from build123d import *

# Parameters (mm, degrees)
ESQUISSE1_W        = 149.75
ESQUISSE1_H        = 135
ESQUISSE1_R        = 1.75
ESQUISSE1_W_2      = 45.5
ESQUISSE1_H_2      = 24.5
BOSS_EXTRU_1_DEPTH = 3
CONG_1_R           = 5
CONG_2_R           = 1


with BuildPart() as part:
    # Esquisse1 → Boss.-Extru.1 (new body)
    with BuildSketch(Plane.XY):
        Rectangle(ESQUISSE1_W, ESQUISSE1_H)
        with Locations((-70, 62.5)):
            Circle(ESQUISSE1_R, mode=Mode.SUBTRACT)
        with Locations((70, 62.5)):
            Circle(ESQUISSE1_R, mode=Mode.SUBTRACT)
        with Locations((55, -51.5)):
            Circle(ESQUISSE1_R, mode=Mode.SUBTRACT)
        with Locations((-55, -51.5)):
            Circle(ESQUISSE1_R, mode=Mode.SUBTRACT)
        with Locations((-58.458333333, 36)):
            Circle(ESQUISSE1_R, mode=Mode.SUBTRACT)
        with Locations((-14.958333333, 29)):
            Circle(ESQUISSE1_R, mode=Mode.SUBTRACT)
        with Locations((1.958333333, 30.25)):
            Circle(ESQUISSE1_R, mode=Mode.SUBTRACT)
        with Locations((62.458333333, 30.25)):
            Circle(ESQUISSE1_R, mode=Mode.SUBTRACT)
        with Locations((62.458333333, -30.25)):
            Circle(ESQUISSE1_R, mode=Mode.SUBTRACT)
        with Locations((1.958333333, -30.25)):
            Circle(ESQUISSE1_R, mode=Mode.SUBTRACT)
        with Locations((-27.75, 17.25)):
            Circle(ESQUISSE1_R, mode=Mode.SUBTRACT)
        with Locations((27.75, 17.25)):
            Circle(ESQUISSE1_R, mode=Mode.SUBTRACT)
        with Locations((27.75, -17.25)):
            Circle(ESQUISSE1_R, mode=Mode.SUBTRACT)
        with Locations((-27.75, -17.25)):
            Circle(ESQUISSE1_R, mode=Mode.SUBTRACT)
        Rectangle(ESQUISSE1_W_2, ESQUISSE1_H_2, mode=Mode.SUBTRACT)
    extrude(amount=BOSS_EXTRU_1_DEPTH)

    # Congé1
    cong_1_edges = [part.edges().sort_by_distance(p)[0] for p in [
        (-74.875, 67.5, 1.5),
        (74.875, 67.5, 1.5),
        (74.875, -67.5, 1.5),
        (-74.875, -67.5, 1.5),
    ]]
    fillet(cong_1_edges, radius=CONG_1_R)

    # Congé2
    cong_2_edges = [part.edges().sort_by_distance(p)[0] for p in [
        (-22.75, 12.25, 1.5),
        (-22.75, -12.25, 1.5),
        (22.75, -12.25, 1.5),
        (22.75, 12.25, 1.5),
    ]]
    fillet(cong_2_edges, radius=CONG_2_R)


solid = part.part
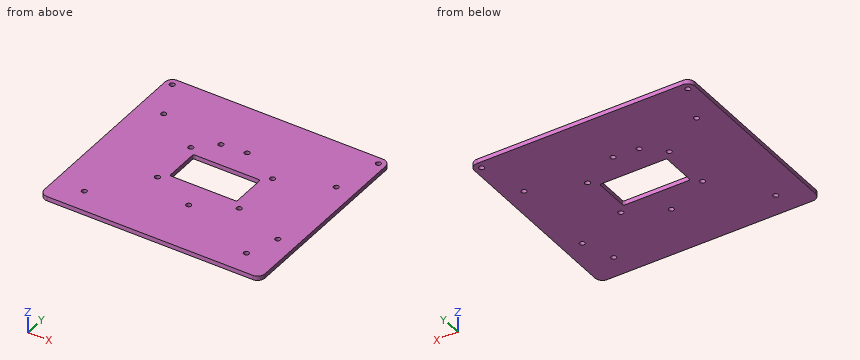
Input: part model. Units: mm. Frame: model coordinates. Round coordinates to 2 decimals unless told otherwise and drop trailing zeros. Order: outer loops, then holes, each group sorted by start corner. A loop starts at its lowest first (then second) coordinate and runs counter-clockwise, first axis right, second up. Notation, with made-up numbers: (-30, -29.5) - (26, -29.5) arc R16 ccw to (26, -15.5) - close; hole circle Ø6 at (-4.75, 84). An arc over 180 degrees is marked (long way). Answer as a JSON object with one key per item and string values. Group by question number.
(1) Cut plane A-A (x = 27.75). Return loops of the section in (y, z), then the cut area to 3 significant figures.
(2) Cut plane C-C (y = -51.5). Return loops of the section in (x, z) (3 decimals), then the cut area to 3 significant figures.
(3) Cut plane B-B (x = 55). Return loops of the section in (y, z), then the cut area to 4 significant figures.
(4) Cut plane D-D (z = 0.7). Count the separate pieces of the cut face and the enclosed holes in it, then the cut area to 3 significant figures.
(5) Material intervals for probe 1 along Y at (x, z) = (-27.75, 1.55); probe 2 along Y at (x, z) = (-70, 2.4); probe 3 along Y at (x, z) = (-55, 0.8), sorted ascending. Write a range as from..to.
Here are the results:
{
 "1": {"outline": "(-67.5, 0) - (-19, 0) - (-19, 3) - (-67.5, 3) - close; (-15.5, 0) - (15.5, 0) - (15.5, 3) - (-15.5, 3) - close; (19, 0) - (67.5, 0) - (67.5, 3) - (19, 3) - close", "area": "384 mm^2"},
 "2": {"outline": "(-74.875, 0) - (-56.75, 0) - (-56.75, 3) - (-74.875, 3) - close; (-53.25, 0) - (53.25, 0) - (53.25, 3) - (-53.25, 3) - close; (56.75, 0) - (74.875, 0) - (74.875, 3) - (56.75, 3) - close", "area": "428 mm^2"},
 "3": {"outline": "(-67.5, 0) - (-53.25, 0) - (-53.25, 3) - (-67.5, 3) - close; (-49.75, 0) - (67.5, 0) - (67.5, 3) - (-49.75, 3) - close", "area": "394.5 mm^2"},
 "4": {"separate pieces": "1", "enclosed holes": "15", "area": "18,900 mm^2"},
 "5": {"probe 1": "y = -67.5..-19, -15.5..15.5, 19..67.5", "probe 2": "y = -67.5..60.75, 64.25..67.5", "probe 3": "y = -67.5..-53.25, -49.75..67.5"}
}
